Input: part model. Units: mm. Frame: model coordinates. Round coordinates to 2 decimals unless told otherwise and drop trailing zeros. Loops run counter-clockwise (first coordinate to the right, second up) from the corner with the lowest first, then second, coordinate; pieces in that order, holes last. Notation, with made-up numbers: (-23.75, 16.25) - (31.25, 16.25) arc R14 ccw to (31.25, 43.25) - close; hole circle Ø9 at (-6.5, 67). An arc over 180 degrees is marked (long way). Write each question's results on one line, items separated by ' | '.
from build123d import *

# Parameters (mm, degrees)
SKETCH1_R           = 122
SKETCH1_R_2         = 120.5
BOSS_EXTRUDE1_DEPTH = 10
BOSS_EXTRUDE2_DEPTH = 30
CIRPATTERN1_COUNT   = 12
SKETCH4_R           = 122
SKETCH4_R_2         = 120.5
BOSS_EXTRUDE3_DEPTH = 10
SKETCH6_W           = 2
SKETCH6_H           = 219.273801444
BOSS_EXTRUDE4_DEPTH = 10
CIRPATTERN2_COUNT   = 4


with BuildPart() as part:
    # Sketch1 → Boss-Extrude1 (new body)
    with BuildSketch(Plane(origin=(0, 0, 0), x_dir=(1, 0, 0), z_dir=(0, 1, 0))):
        Circle(SKETCH1_R)
        Circle(SKETCH1_R_2, mode=Mode.SUBTRACT)
    extrude(amount=BOSS_EXTRUDE1_DEPTH)

    # Sketch3 → Boss-Extrude2 (add)
    with BuildSketch(Plane(origin=(0, 10, 0), x_dir=(1, 0, 0), z_dir=(0, 1, 0))):
        with BuildLine():
            Line((34.717842259, 115.390300411), (34.717842259, 116.955852478))
            ThreePointArc((34.717842259, 116.955852478), (32.225116431, 117.66708066), (29.717842259, 118.325186885))
            Line((29.717842259, 118.325186885), (29.717842259, 116.777993866))
            ThreePointArc((29.717842259, 116.777993866), (32.22531277, 116.111064145), (34.717842259, 115.390300411))
        make_face()
    boss_extrude2 = extrude(amount=BOSS_EXTRUDE2_DEPTH)

    # CirPattern1: Boss-Extrude2 ×12 about axis
    cirpattern1_axis = Axis((0, 0, 0), (0, 1, 0))
    for i in range(1, CIRPATTERN1_COUNT):
        add(boss_extrude2.rotate(cirpattern1_axis, i * 360 / CIRPATTERN1_COUNT))

    # Sketch4 → Boss-Extrude3 (add)
    with BuildSketch(Plane(origin=(0, 40, 0), x_dir=(1, 0, 0), z_dir=(0, 1, 0))):
        Circle(SKETCH4_R)
        Circle(SKETCH4_R_2, mode=Mode.SUBTRACT)
    extrude(amount=BOSS_EXTRUDE3_DEPTH)

    # Sketch6 → Boss-Extrude4 (add)
    with BuildSketch(Plane(origin=(0, 0, 0), x_dir=(1, 0, 0), z_dir=(0, 1, 0))):
        with Locations((-51, 0)):
            Rectangle(SKETCH6_W, SKETCH6_H)
    boss_extrude4 = extrude(amount=BOSS_EXTRUDE4_DEPTH)

    # CirPattern2: Boss-Extrude4 ×4 about axis
    cirpattern2_axis = Axis((0, 0, 0), (0, 1, 0))
    for i in range(1, CIRPATTERN2_COUNT):
        add(boss_extrude4.rotate(cirpattern2_axis, i * 360 / CIRPATTERN2_COUNT))


solid = part.part
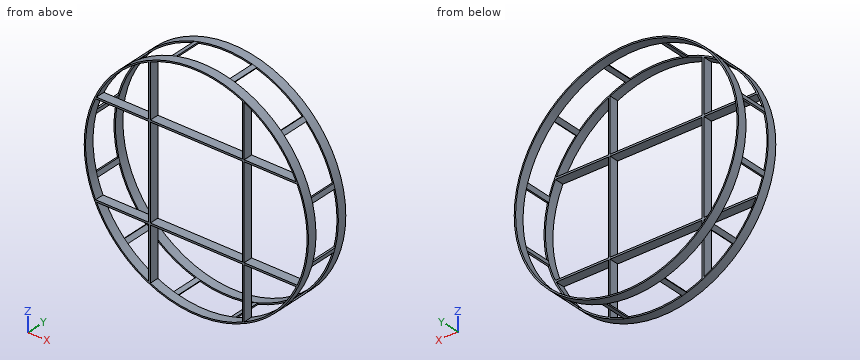
1. Section query A-A, the plane z = 0. Output: boundary loops of the cut face in (x, y).
Answer:
outline: (-122, 0) - (-120.5, 0) - (-120.5, 10) - (-122, 10) - close; (-122, 40) - (-120.5, 40) - (-120.5, 50) - (-122, 50) - close; (-52, 0) - (-50, 0) - (-50, 10) - (-52, 10) - close; (50, 0) - (52, 0) - (52, 10) - (50, 10) - close; (120.5, 0) - (122, 0) - (122, 10) - (120.5, 10) - close; (120.5, 40) - (122, 40) - (122, 50) - (120.5, 50) - close
2. Section query B-B, the plane x = 0. Output: boundary loops of the cut face in (y, z), plus the area to 3 significant figures.
Answer:
outline: (0, -122) - (10, -122) - (10, -120.5) - (0, -120.5) - close; (0, -52) - (10, -52) - (10, -50) - (0, -50) - close; (0, 50) - (10, 50) - (10, 52) - (0, 52) - close; (0, 120.5) - (10, 120.5) - (10, 122) - (0, 122) - close; (40, -122) - (50, -122) - (50, -120.5) - (40, -120.5) - close; (40, 120.5) - (50, 120.5) - (50, 122) - (40, 122) - close | area: 100 mm^2
3. Line query: line 1 (Z direction, x = 0, y = 43.5); line 2 (X direction, y = 7, z = 73.5). Output: solid intervals per line, ascending. Write a range as [from, to].
Answer:
line 1: [-122, -120.5], [120.5, 122] | line 2: [-97.37, -95.49], [-52, -50], [50, 52], [95.49, 97.37]
4. Section query C-C, the plane y = 7. Count the separate pieces of the cut face and the enclosed holes in it, plus the area to 3 significant figures.
Answer:
separate pieces: 1 | enclosed holes: 9 | area: 2,870 mm^2
5. Contact query for flat-ended pins moving along their axis: pin 1 (10 mm diameter, centred on y = 11, z = 80.5, fed in from +X); pin 2 (8 mm diameter, centred on x = 38, y = 21.5, fed in from -Z); pin 3 (8 mm diameter, centred on x = 5.5, y = 6, fed in from +Z). Output: stop coordinate, or through.
Answer:
pin 1: x = 95.75 | pin 2: z = -117.17 | pin 3: z = 121.99
